Source: three-view drawing plus pictorial views. Frame: mm from the lowest corner of the part. A direction names the side the tool comes from. Give positions to 0.01 mm unless a question says otherwise; leave off trailing zeros. Loops run counter-clockwise (first coordinate to the right, second up) from the corner with the lowest first, then second, coordinate; pieces in that order, holes last. Notation, with made-up numbers: (0.5, 59.25) -> (8.5, 59.25) arc R31 ccw to (8.5, 95.25) -> close; hole circle Ø10 at (88.5, 74.5). An arc over 180 degrees is marked (long way). Answer in a Markdown table with one row per item. Add a question column.
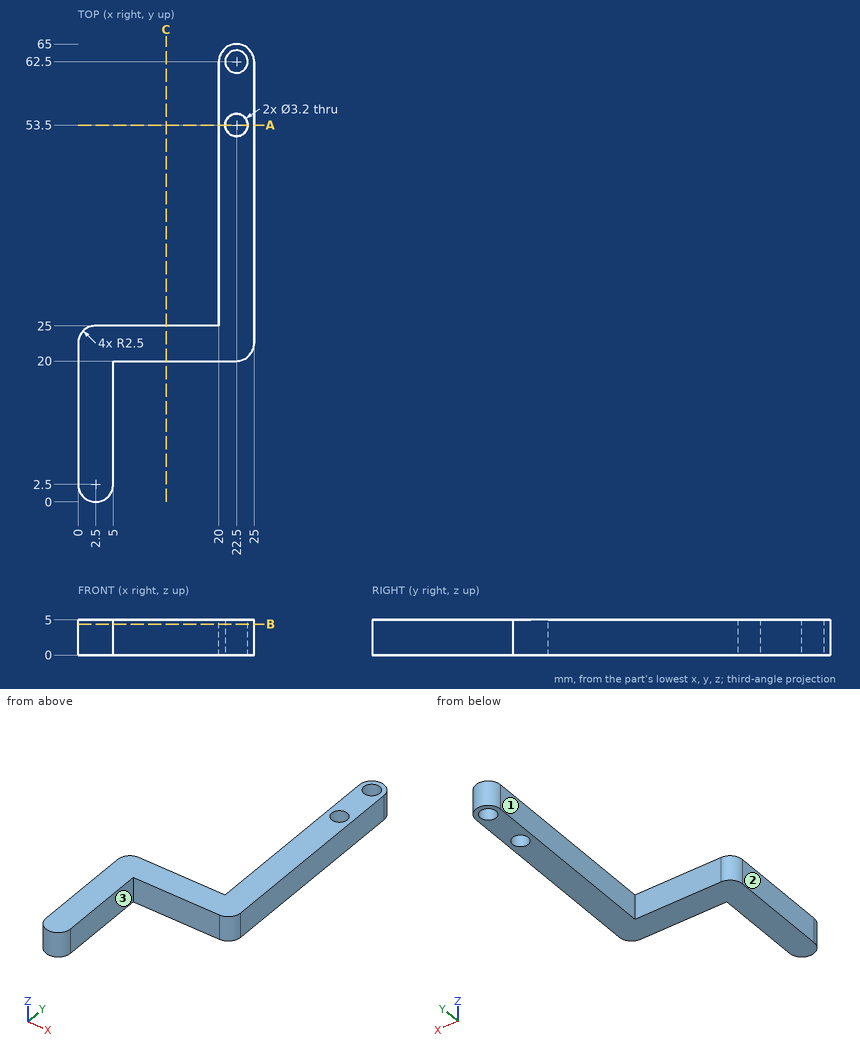
(1) Pin query (flat end, axial travel): pin 1 Ø2.5 at (x, z) = (15, 3) entering from +Y; pin 2 Ø1.5 at (x, z) = (19.5, 4) entering from -Y. Return the tip coordinate at first contact, or that it passes through.
(2) Material intervals for line 1 along Y through (x, z) = (22.5, 3.4); line 2 along Y through (x, z) = (23, 0.75); line 3 along X through (y, z) = (53.5, 2.05), sorted ascending. Write a range as from..to.
(3) Cut plane C-C on x = 12.5. Return the cut outline in (y, z).
(4) Cut plane A-A on y = 53.5. Return the cut outline in (x, z).
(5) Cut plane B-B on z = 4.4. Return the cut outline in (x, y).
(6) Reachability of the marked faces 1, 2 and 3 from +Z, -Z, +X, -X, +Y, -Y: full face, straight path, thin tool, end or side. Return the list, or none.
Answer list:
| question | item | result |
|---|---|---|
| 1 | pin 1 | stops at y = 25 |
| 1 | pin 2 | stops at y = 20 |
| 2 | line 1 | y = 20..51.9, 55.1..60.9, 64.1..65 |
| 2 | line 2 | y = 20.05..51.98, 55.02..60.98, 64.02..64.95 |
| 2 | line 3 | x = 20..20.9, 24.1..25 |
| 3 | outline | (20, 0) -> (25, 0) -> (25, 5) -> (20, 5) -> close |
| 4 | outline | (20, 0) -> (20.9, 0) -> (20.9, 5) -> (20, 5) -> close; (24.1, 0) -> (25, 0) -> (25, 5) -> (24.1, 5) -> close |
| 5 | outline | (0, 2.5) arc R2.5 ccw to (5, 2.5) -> (5, 20) -> (22.5, 20) arc R2.5 ccw to (25, 22.5) -> (25, 62.5) arc R2.5 ccw to (20, 62.5) -> (20, 25) -> (2.5, 25) arc R2.5 ccw to (0, 22.5) -> close; hole circle Ø3.2 at (22.5, 53.5); hole circle Ø3.2 at (22.5, 62.5) |
| 6 | face 1 | +Z, -Z, -X, +Y |
| 6 | face 2 | +Z, -Z, -X, +Y, -Y |
| 6 | face 3 | +Z, -Z, +X, -Y |
